Here's how the part is built. I have some questions about the finished solid (model axes, mm). Face numbers are marked on the shaded views. Round coordinates to 2 decimals unless told otherwise and drop trailing zeros. Write each loop counter-clockwise with the first axis right and the second up, starting at its lowest first coordinate (ties: lowest second). Pieces come first, ordered by that corner, then holes. Notation, with made-up numbers: (51.5, 44) -> (101.5, 44) arc R26 ccw to (101.5, 60) -> close; hole circle Ø11 at (-22, 63.5). An arc over 180 degrees is marked (long way). Answer as CSV lines item,"result".
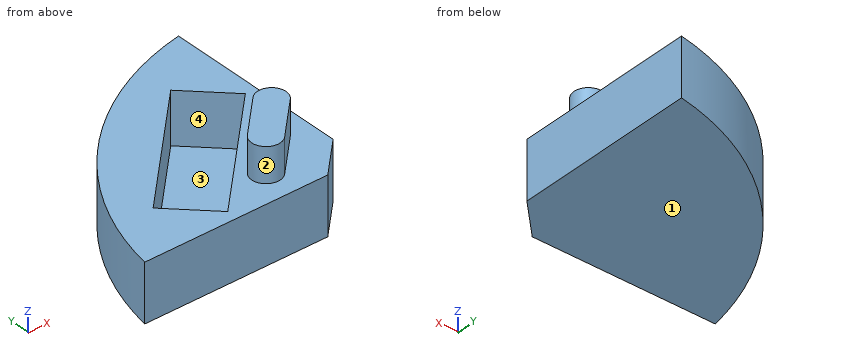
from build123d import *

# Parameters (mm, degrees)
F1_DEPTH = 5
F3_DEPTH = 4.5
F5_DEPTH = 3


with BuildPart() as f1:
    # F0 (on Top) → F1 (new body)
    with BuildSketch(Plane.XY):
        with BuildLine():
            Line((-3, 0), (0, 3))
            Line((0, 3), (0, 19))
            ThreePointArc((0, 19), (-12.510187, 12.510187), (-19, 0))
            Line((-19, 0), (-3, 0))
        make_face()
    extrude(amount=F1_DEPTH)

    # F2 (on face) → F3 (cut)
    with BuildSketch(Plane.XY.offset(5)):
        Polygon((-10.899495, 1), (-1, 10.899495), (-4.535534, 14.435029), (-14.435029, 4.535534), align=None)
    extrude(amount=-F3_DEPTH, mode=Mode.SUBTRACT)

    # F4 (on face) → F5 (join)
    with BuildSketch(Plane.XY.offset(5)):
        with BuildLine():
            Line((-3.713925, 6.892677), (-6.895905, 3.710697))
            ThreePointArc((-6.895905, 3.710697), (-6.895098, 1.942122), (-5.126524, 1.944544))
            Line((-5.126524, 1.944544), (-1.944544, 5.126524))
            ThreePointArc((-1.944544, 5.126524), (-1.945351, 6.895099), (-3.713925, 6.892677))
        make_face()
    extrude(amount=F5_DEPTH)


solid = f1.part
Item 1: Suppose I cut it at D-D, the plane z = 7.75. List the corners of the cut face in (x, y) for me.
Results found:
outline,"(-6.9, 3.71) arc R1.25 ccw to (-5.13, 1.94) -> (-1.94, 5.13) arc R1.25 ccw to (-3.71, 6.89) -> close"
Item 2: Suppose I cut it at B-B, the plane x = -11.75. List the corners of the cut face in (y, z) for me, then the cut area to 3 significant figures.
Results found:
outline,"(0, 0) -> (13.24, 0) -> (13.24, 5) -> (7.22, 5) -> (7.22, 0.5) -> (1.85, 0.5) -> (1.85, 5) -> (0, 5) -> close"
area,"42.0 mm²"
Item 3: I need wall thicknesses on L1, parallel to Z at x = -3, y = 10; L2, parallel to Z at x = -9, y = 2; L3, parallel to Y at x = -12.5, z = 1.25. Which ranges of each line are inside material? Lowest first, please.
Results found:
L1,"z = 0 to 0.5"
L2,"z = 0 to 5"
L3,"y = 0 to 2.6, 6.47 to 12.52"
Item 4: Will this pin go through, and if not, where does the flat tip stop? pin 1 (2 mm diameter, centred on x = -6, y = 9.5, fed in from +Z).
Results found:
pin 1,"stops at z = 0.5"
Item 5: Suppose I cut it at C-C, the plane y = 6.25. List the corners of the cut face in (x, z) for me, then the cut area to 3 significant figures.
Results found:
outline,"(-16.98, 0) -> (0, 0) -> (0, 5) -> (-1.6, 5) -> (-1.6, 8) -> (-4.36, 8) -> (-4.36, 5) -> (-5.65, 5) -> (-5.65, 0.5) -> (-12.72, 0.5) -> (-12.72, 5) -> (-16.98, 5) -> close"
area,"61.3 mm²"
Item 6: Suppose I cut it at A-A, the plane z = 2.75. List the corners of the cut face in (x, y) for me, then the cut area to 3 significant figures.
Results found:
outline,"(-19, 0) -> (-3, 0) -> (0, 3) -> (0, 19) arc R23.33 ccw to start; hole (-14.44, 4.54) -> (-10.9, 1) -> (-1, 10.9) -> (-4.54, 14.44) -> close"
area,"184 mm²"
Item 7: If we mould it in two halves opening along Y, with no side actions, what happens to the marked faces 1, 2, 3 and 4? For each: pulls with the +Y half, pulls with the -Y half, needs draft (parallel to the pull), parting line crosses it, or undercut.
Results found:
face 1,"needs draft"
face 2,"parting line crosses it"
face 3,"undercut"
face 4,"undercut"
